Can you work these out from the drawing? Everything is in mm from the part's minimum corner. A direction names the side the tool comes from. Coordinates: 2 decimals unless noted, no trailing zeros. Order: outer loops, then holes, each group sorted by start corner. A loop starts at its lowest first (then second) coordinate and runs counter-clockwise, first axis right, second up. Notation, with made-up numbers: (9, 59) - (54, 59) arc R5 ccw to (54, 64) - close; hole circle Ø3 at (-14.5, 11.5). An arc over 180 degrees is marked (long way). One line per item, written item: value.
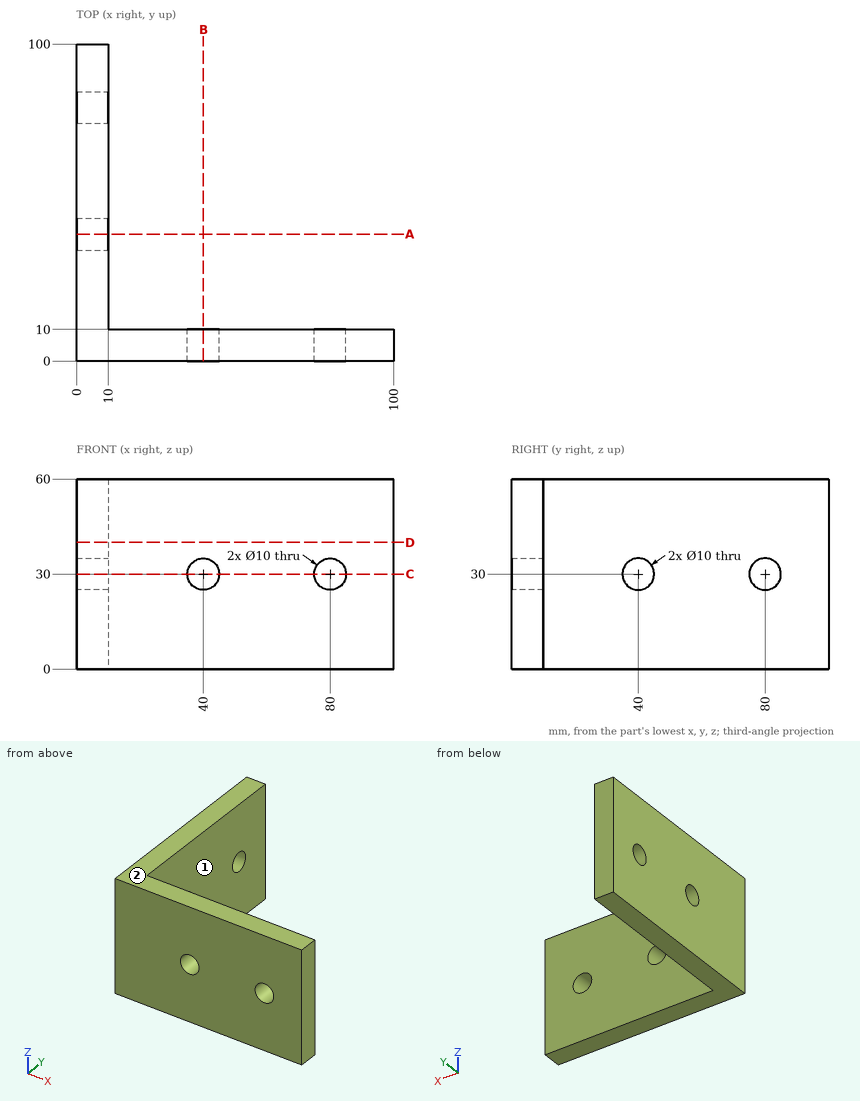
Item 1: I'm going to push flat-ended pins straight in: pin 1 Ø3 at (x, z) = (28.5, 21.5) entering from +Y; pin 2 Ø1.5 at (y, z) = (89, 35) entering from +X; pin 3 Ø13 at (y, z) = (80, 30) entering from -X. Where does each tip first touch, or does it pass through?
Conclusion:
pin 1: y = 10
pin 2: x = 10
pin 3: x = 0
Item 2: I want a section at D-D on z = 40. Please give me the cut outline in (x, y).
Conclusion:
outline: (0, 0) - (100, 0) - (100, 10) - (10, 10) - (10, 100) - (0, 100) - close
Item 3: For the marked faces 1 and 2, which set-ups out of +Z, -Z, +X, -X, +Y, -Y let a thin tool reach every point of the face, with its end or its side?
Conclusion:
face 1: +Z, -Z, +X, +Y
face 2: +Z, +X, -X, +Y, -Y
Item 4: I want a section at A-A on y = 40. Please give me the cut outline in (x, z), then the cut area to 3 significant figures.
Conclusion:
outline: (0, 0) - (10, 0) - (10, 25) - (0, 25) - close; (0, 35) - (10, 35) - (10, 60) - (0, 60) - close
area: 500 mm²
Item 5: I want a section at C-C on z = 30. Please give me the cut outline in (x, y).
Conclusion:
outline: (0, 0) - (35, 0) - (35, 10) - (10, 10) - (10, 35) - (0, 35) - close; (0, 45) - (10, 45) - (10, 75) - (0, 75) - close; (0, 85) - (10, 85) - (10, 100) - (0, 100) - close; (45, 0) - (75, 0) - (75, 10) - (45, 10) - close; (85, 0) - (100, 0) - (100, 10) - (85, 10) - close
Item 6: If I drill on probe 1 along Y at (x, z) = (5, 30); probe 2 along Z at (x, y) = (40, 8), over which ranges is the centre line in solid material (lowest first)?
Conclusion:
probe 1: 0 to 35, 45 to 75, 85 to 100
probe 2: 0 to 25, 35 to 60
